from build123d import *

# Parameters (mm, degrees)
BOSS_EXTRUDE1_DEPTH      = 4
CROQUIS3_W               = 75
CROQUIS3_H               = 20
CORTAR_EXTRUIR1_DEPTH    = 10
CROQUIS4_R               = 3.5
SALIENTE_EXTRUIR1_DEPTH  = 2
CROQUIS5_R               = 2.5
SALIENTE_EXTRUIR2_DEPTH  = 27
CORTAR_EXTRUIR3_DEPTH    = 171.194006945
REDONDEO2_R              = 2
REDONDEO3_R              = 2
REDONDEO4_R              = 2
REDONDEO5_R              = 2
REDONDEO6_R              = 2
REDONDEO7_R              = 10
CROQUIS9_R               = 1.5
CORTAR_EXTRUIR4_DEPTH    = 171.194006945
CROQUIS15_R              = 3.75
SALIENTE_EXTRUIR3_DEPTH  = 10
REDONDEO8_R              = 10
REDONDEO8_OF_SIMETR_A2_R = 10
CROQUIS16_W              = 45.868264646
CROQUIS16_H              = 20
CROQUIS16_W_2            = 25.985344102
CROQUIS16_W_3            = 31
CROQUIS16_W_4            = 32
SALIENTE_EXTRUIR5_DEPTH  = 5


# Some blends are built 0.0001 mm under size
with BuildPart() as part:
    # Sketch1 → Boss-Extrude1 (new body)
    with BuildSketch(Plane(origin=(0, 0, 0), x_dir=(1, 0, 0), z_dir=(0, 1, 0))):
        with BuildLine():
            Line((70, 75), (150, 75))
            Line((150, 75), (150, 65))
            Line((150, 65), (150, -30))
            Line((150, -30), (150, -75))
            Line((150, -75), (70, -75))
            Line((70, -75), (-140, -75))
            ThreePointArc((-140, -75), (-147.071067812, -72.071067812), (-150, -65))
            Line((-150, -65), (-150, 65))
            ThreePointArc((-150, 65), (-147.071067812, 72.071067812), (-140, 75))
            Line((-140, 75), (70, 75))
        make_face()
    extrude(amount=BOSS_EXTRUDE1_DEPTH)

    # Croquis3 → Cortar-Extruir1 (cut)
    with BuildSketch(Plane(origin=(0, 4, 0), x_dir=(1, 0, 0), z_dir=(0, 1, 0))):
        with Locations((-102.5, 65)):
            Rectangle(CROQUIS3_W, CROQUIS3_H)
        with Locations((-102.5, -65)):
            Rectangle(CROQUIS3_W, CROQUIS3_H)
        Polygon((47.925951559, -36.159033642), (16.439774713, -75), (143.560225287, -75), (112.074048441, -36.159033642), (102.074048441, -36.159033642), (85, -50), (75, -50), (57.925951559, -36.159033642), align=None)
        Polygon((143.560225287, 75), (16.439774713, 75), (47.925951559, 36.159033642), (57.925951559, 36.159033642), (75, 50), (85, 50), (102.074048441, 36.159033642), (112.074048441, 36.159033642), align=None)
    cortar_extruir1 = extrude(amount=-CORTAR_EXTRUIR1_DEPTH, mode=Mode.SUBTRACT)

    # Croquis4 → Saliente-Extruir1 (add)
    with BuildSketch(Plane(origin=(0, 4, 0), x_dir=(1, 0, 0), z_dir=(0, 1, 0))):
        with Locations(Location((80, 42, 0), (0, 0, 270))):
            Circle(CROQUIS4_R)
        with Locations(Location((80, -42, 0), (0, 0, 90))):
            Circle(CROQUIS4_R)
    extrude(amount=SALIENTE_EXTRUIR1_DEPTH)

    # Croquis5 → Saliente-Extruir2 (add)
    with BuildSketch(Plane(origin=(0, 6, 0), x_dir=(1, 0, 0), z_dir=(0, 1, 0))):
        with Locations(Location((80, 42, 0), (0, 0, 270))):
            Circle(CROQUIS5_R)
        with Locations(Location((80, -42, 0), (0, 0, 90))):
            Circle(CROQUIS5_R)
    extrude(amount=SALIENTE_EXTRUIR2_DEPTH)

    # Croquis7 → Cortar-Extruir3 (cut, through all)
    with BuildSketch(Plane(origin=(0, 4, 0), x_dir=(1, 0, 0), z_dir=(0, 1, 0))):
        Polygon((57.925951559, 36.159033642), (48.662122101, 28.38575776), (40.074307196, 28.38575776), (16.439774713, 75), align=None)
        Polygon((16.439774713, -75), (57.925951559, -36.159033642), (48.662122101, -28.38575776), (40.074307196, -28.38575776), align=None)
        Polygon((143.560225287, 75), (102.074048441, 36.159033642), (111.337877899, 28.38575776), (119.925692804, 28.38575776), align=None)
        Polygon((102.074048441, -36.159033642), (111.337877899, -28.38575776), (119.925692804, -28.38575776), (143.560225287, -75), align=None)
    extrude(amount=-CORTAR_EXTRUIR3_DEPTH, mode=Mode.SUBTRACT)

    # Redondeo2
    redondeo2_edges = [part.edges().sort_by_distance(p)[0] for p in [
        (80, 4, -45.5),
    ]]
    fillet(redondeo2_edges, radius=REDONDEO2_R - 0.0001)  # a hair under: the kernel refuses the full size

    # Redondeo3
    # the kernel refuses this fillet: 2 mm, written as the material it adds along each edge
    with BuildSketch(Plane(origin=(80, 6, -42), x_dir=(0, 0, 1), z_dir=(-1, 0, 0))) as redondeo3_piece_1:
        with BuildLine():
            CenterArc((4.5, 1.732050808), REDONDEO3_R, 180, 60)
            Line((2.5, 1.732050808), (2.46, 1.732050808))
            Line((2.46, 1.732050808), (2.46, 0))
            Line((2.46, 0), (2.5, -0.04))
            ThreePointArc((2.5, -0.04), (3, -0.04), (3.48, -0.034641016))
            Line((3.48, -0.034641016), (3.5, 0))
        make_face()
    revolve(axis=Axis((80, 6, -42), (0, 1, 0)))

    # Redondeo4
    redondeo4_edges = [part.edges().sort_by_distance(p)[0] for p in [
        (80, 6, -45.5),
    ]]
    fillet(redondeo4_edges, radius=REDONDEO4_R)

    # Redondeo5
    # the kernel refuses this fillet: 2 mm, written as the material it adds along each edge
    with BuildSketch(Plane(origin=(80, 4, 42), x_dir=(0, 0, -1), z_dir=(1, 0, 0))) as redondeo5_piece_1:
        with BuildLine():
            CenterArc((3.5 + REDONDEO5_R, REDONDEO5_R), REDONDEO5_R, 180, 90)
            Line((3.5, REDONDEO5_R), (3.5 - REDONDEO5_R * 0.02, REDONDEO5_R))
            Line((3.5 - REDONDEO5_R * 0.02, REDONDEO5_R), (3.5 - REDONDEO5_R * 0.02, -REDONDEO5_R * 0.02))
            Line((3.5 - REDONDEO5_R * 0.02, -REDONDEO5_R * 0.02), (3.5 + REDONDEO5_R, -REDONDEO5_R * 0.02))
            Line((3.5 + REDONDEO5_R, -REDONDEO5_R * 0.02), (3.5 + REDONDEO5_R, 0))
        make_face()
    revolve(axis=Axis((80, 4, 42), (0, 1, 0)))
    with BuildSketch(Plane(origin=(80, 6, 42), x_dir=(0, 0, -1), z_dir=(1, 0, 0))) as redondeo5_piece_2:
        with BuildLine():
            CenterArc((4.5, 1.732050808), REDONDEO5_R, 180, 60)
            Line((2.5, 1.732050808), (2.46, 1.732050808))
            Line((2.46, 1.732050808), (2.46, 0))
            Line((2.46, 0), (2.5, -0.04))
            ThreePointArc((2.5, -0.04), (3, -0.04), (3.48, -0.034641016))
            Line((3.48, -0.034641016), (3.5, 0))
        make_face()
    revolve(axis=Axis((80, 6, 42), (0, 1, 0)))

    # Redondeo6
    redondeo6_edges = [part.edges().sort_by_distance(p)[0] for p in [
        (80, 6, 45.5),
    ]]
    fillet(redondeo6_edges, radius=REDONDEO6_R)

    # Redondeo7
    # the kernel refuses this fillet: 10 mm, written as the material it adds along each edge
    with BuildSketch(Plane(origin=(40.074307196, 4, 28.38575776), x_dir=(-0.4522182722164984, 0, 0.8919073013904107), z_dir=(0, -1, 0)), Plane(origin=(119.925692804, 4, 28.38575776), x_dir=(-1, 0, 0), z_dir=(0, -1, 0))) as redondeo7_piece_1:
        with BuildLine():
            CenterArc((REDONDEO7_R * 0.614168901779, -REDONDEO7_R), REDONDEO7_R, 90, 63.113904691)
            Line((-REDONDEO7_R * 0.277738399612, -REDONDEO7_R * 0.547781727784), (0, 0))
            Line((0, 0), (REDONDEO7_R * 0.614168901779, 0))
        make_face()
    extrude(amount=4)
    with BuildSketch(Plane(origin=(48.662122101, 4, 28.38575776), x_dir=(-1, 0, 0), z_dir=(0, -1, 0)), Plane(origin=(111.337877899, 4, 28.38575776), x_dir=(-0.7660444431189768, 0, 0.6427876096865409), z_dir=(0, -1, 0))) as redondeo7_piece_2:
        with BuildLine():
            CenterArc((REDONDEO7_R * 0.363970234266, -REDONDEO7_R), REDONDEO7_R, 90, 40)
            Line((-REDONDEO7_R * 0.27881737542, -REDONDEO7_R * 0.233955556881), (0, 0))
            Line((0, 0), (REDONDEO7_R * 0.363970234266, 0))
        make_face()
    extrude(amount=4)
    with BuildSketch(Plane(origin=(40.074307196, 4, -28.38575776), x_dir=(-0.4522182722164984, 0, -0.8919073013904107), z_dir=(0, -1, 0)), Plane(origin=(119.925692804, 4, -28.38575776), x_dir=(-1, 0, 0), z_dir=(0, -1, 0))) as redondeo7_piece_3:
        with BuildLine():
            CenterArc((REDONDEO7_R * 0.614168901779, REDONDEO7_R), REDONDEO7_R, 206.886095309, 63.113904691)
            Line((-REDONDEO7_R * 0.277738399612, REDONDEO7_R * 0.547781727784), (0, 0))
            Line((0, 0), (REDONDEO7_R * 0.614168901779, 0))
        make_face()
    extrude(amount=4)
    with BuildSketch(Plane(origin=(48.662122101, 4, -28.38575776), x_dir=(-1, 0, 0), z_dir=(0, -1, 0)), Plane(origin=(111.337877899, 4, -28.38575776), x_dir=(-0.7660444431189768, 0, -0.6427876096865409), z_dir=(0, -1, 0))) as redondeo7_piece_4:
        with BuildLine():
            CenterArc((REDONDEO7_R * 0.363970234266, REDONDEO7_R), REDONDEO7_R, 230, 40)
            Line((-REDONDEO7_R * 0.27881737542, REDONDEO7_R * 0.233955556881), (0, 0))
            Line((0, 0), (REDONDEO7_R * 0.363970234266, 0))
        make_face()
    extrude(amount=4)

    # Croquis9 → Cortar-Extruir4 (cut, through all)
    with BuildSketch(Plane(origin=(0, 4, 0), x_dir=(1, 0, 0), z_dir=(0, 1, 0))):
        with Locations(Location((-107.59, 25.23, 0), (0, 0, 270))):
            Circle(CROQUIS9_R)
        with Locations(Location((-79.79, 25.33, 0), (0, 0, 270))):
            Circle(CROQUIS9_R)
        with Locations(Location((-79.79, -22.45, 0), (0, 0, 270))):
            Circle(CROQUIS9_R)
        with Locations(Location((-107.59, -22.57, 0), (0, 0, 270))):
            Circle(CROQUIS9_R)
    extrude(amount=-CORTAR_EXTRUIR4_DEPTH, mode=Mode.SUBTRACT)

    # Croquis15 → Saliente-Extruir3 (add)
    with BuildSketch(Plane(origin=(0, 0, -55), x_dir=(-1, 0, 0), z_dir=(0, 0, -1))):
        with BuildLine():
            Line((89.459684655, 4), (89.459684655, 18.25))
            ThreePointArc((89.459684655, 18.25), (102.19671333, 30.27014077), (113.459684655, 16.858908145))
            Line((113.459684655, 16.858908145), (113.459684655, 4))
            Line((113.459684655, 4), (89.459684655, 4))
        make_face()
        with Locations((101.5, 18.25)):
            Circle(CROQUIS15_R, mode=Mode.SUBTRACT)
    saliente_extruir3 = extrude(amount=-SALIENTE_EXTRUIR3_DEPTH)

    # Redondeo8
    redondeo8_edges = [part.edges().sort_by_distance(p)[0] for p in [
        (-113.459684655, 4, -50),
        (-89.459684655, 4, -50),
        (-101.459684655, 4, -45),
    ]]
    fillet(redondeo8_edges, radius=REDONDEO8_R)

    # Simetría2: Cortar-Extruir1, Saliente-Extruir3 across plane
    add(cortar_extruir1.mirror(Plane.XY), mode=Mode.SUBTRACT)
    add(saliente_extruir3.mirror(Plane.XY))

    # Redondeo8 of Simetría2
    redondeo8_of_simetr_a2_edges = [part.edges().sort_by_distance(p)[0] for p in [
        (-113.459684655, 4, 50),
        (-89.459684655, 4, 50),
        (-101.459684655, 4, 45),
    ]]
    fillet(redondeo8_of_simetr_a2_edges, radius=REDONDEO8_OF_SIMETR_A2_R)

    # Croquis16 → Saliente-Extruir5 (add)
    with BuildSketch(Plane.XZ):
        Polygon((-94.131735354, 47.5), (-94.131735354, 14), (-140, 14), (-140, 47.5), (-144, 47.5), (-144, -47.5), (-140, -47.5), (-140, -14), (-94.131735354, -14), (-94.131735354, -47.5), (-90.131735354, -47.5), (-90.131735354, -14), (-44.263470708, -14), (-44.263470708, -47.5), (-40.263470708, -47.5), (-40.263470708, -14), (5.604793938, -14), (5.604793938, -47.5), (9.604793938, -47.5), (9.604793938, -14), (40.604793938, -14), (40.604793938, -22.5), (44.604793938, -22.5), (44.604793938, -14), (76.604793938, -14), (76.604793938, -22.5), (80.604793938, -22.5), (80.604793938, -14), (112.604793938, -14), (112.604793938, -22.5), (116.604793938, -22.5), (116.604793938, -14), (142.59013804, -14), (142.59013804, -67.5), (146.59013804, -67.5), (146.59013804, -14), (146.59013804, 10), (146.59013804, 14), (146.59013804, 67.5), (142.59013804, 67.5), (142.59013804, 14), (116.604793938, 14), (116.604793938, 22.5), (112.604793938, 22.5), (112.604793938, 14), (80.604793938, 14), (80.604793938, 22.5), (76.604793938, 22.5), (76.604793938, 14), (44.604793938, 14), (44.604793938, 22.5), (40.604793938, 22.5), (40.604793938, 14), (9.604793938, 14), (9.604793938, 47.5), (5.604793938, 47.5), (5.604793938, 14), (-40.263470708, 14), (-40.263470708, 47.5), (-44.263470708, 47.5), (-44.263470708, 14), (-90.131735354, 14), (-90.131735354, 47.5), align=None)
        with Locations((-117.065867677, 0)):
            Rectangle(CROQUIS16_W, CROQUIS16_H, mode=Mode.SUBTRACT)
        with Locations((129.597465989, 0)):
            Rectangle(CROQUIS16_W_2, CROQUIS16_H, mode=Mode.SUBTRACT)
        with Locations((25.104793938, 0)):
            Rectangle(CROQUIS16_W_3, CROQUIS16_H, mode=Mode.SUBTRACT)
        with Locations((60.604793938, 0)):
            Rectangle(CROQUIS16_W_4, CROQUIS16_H, mode=Mode.SUBTRACT)
        with Locations((96.604793938, 0)):
            Rectangle(CROQUIS16_W_4, CROQUIS16_H, mode=Mode.SUBTRACT)
        with Locations((-17.329338385, 0)):
            Rectangle(CROQUIS16_W, CROQUIS16_H, mode=Mode.SUBTRACT)
        with Locations((-67.197603031, 0)):
            Rectangle(CROQUIS16_W, CROQUIS16_H, mode=Mode.SUBTRACT)
    extrude(amount=SALIENTE_EXTRUIR5_DEPTH)


solid = part.part
Design review of the part built by this model. Coordinates are the model's own, in mm. A direction names the side the tool comes from. Round coordinates to 2 decimals unless told otherwise and drop trailing zeros. Write each loop counter-clockwise with the first axis right and the second up, starting at its lowest first coordinate (ties: lowest second). Pieces come first, ordered by that corner, then holes. Notation, with made-up numbers: (40.5, 30) - (69.5, 30) arc R5 ccw to (69.5, 35) - close; hole circle Ø8 at (1, -36.75). An arc over 180 degrees is marked (long way). Return JSON: item names as keys, results as strings. Group by question number.
Item 1: We need section B-B on y = 27.5. Write out the cut boundary in (x, z), and give its area (3 significant figures).
Item 2: The part is to be moulded in two halves that separate along Z. For faces 5 (the face through (-146.99, 1.97, 72.15)), 6 (the face through (96, 0, 0)), 7 (the face through (-104.964, 16.814, -50.07)), 8 (the face through (-117, 0, 0)), say which applies: pulls with the +Z half, pulls with the -Z half, needs draft (parallel to the pull), parting line crosses it, or undercut.
Item 3: For probe 1 along X at (y, z) = (1.4, 22.45); probe 2 along Z at (x, y) = (-79.79, 1.7); probe 3 along Y at (x, z) = (-101, -51), list the stretches that pass through material, from the lowest coordinate up. Write a range as [from, to].
Item 4: We need section A-A on x = -101.5. Write out the cut boundary in (y, z).
Item 5: Machinability: for faces 1 (the face through (-101.7, 22.3, 45)), 2 (the face through (-68, 0, 0)), 3 (the face through (-104.964, 16.814, 50.07)), 4 (the face through (66.34, 2.03, -42.98)), which of the approach directions +Z, -Z, +X, -X, +Y, -Y give a long, thin tool a straight path to every point of the face, cutting with its end or side? Answer none if there is none.
Item 6: We need section C-C on x = -69.5. Write out the cut boundary in (y, z).
Item 7: Insertion check: P1, Ø5, axis at x = 101, z = 38, coming from the +Y side; P2, Ø1.5, axis at x = -117.5, y = -2, coming from the +Z side; P3, Ø5, axis at x = -102.5, y = 7, coming from the +Z side. Each pin has a flat end and moves straight along its axis. Give the tip position at first contact, or say it passes through.
Model answer:
{
 "1": {"outline": "(-109.21, -55) - (-93.79, -55) - (-93.79, -45) - (-109.21, -45) - close; (-109.21, 45) - (-93.79, 45) - (-93.79, 55) - (-109.21, 55) - close; circle Ø5 at (80, -42); circle Ø5 at (80, 42)", "area": "348 mm²"},
 "2": {"face 5": "pulls with the +Z half", "face 6": "undercut", "face 7": "needs draft", "face 8": "undercut"},
 "3": {"probe 1": "x = [-150, -109.09], [-106.09, -81.29], [-78.29, 150]", "probe 2": "z = [-55, -26.83], [-23.83, 20.95], [23.95, 55]", "probe 3": "y = [0, 14.53], [21.97, 30.28]"},
 "4": {"outline": "(-5, -14) - (0, -14) - (0, -55) - (14.5, -55) - (14.5, -45) - (14, -45) arc R10 cw to (4, -35) - (4, 35) arc R10 cw to (14, 45) - (14.5, 45) - (14.5, 55) - (0, 55) - (0, 14) - (-5, 14) - (-5, 10) - (0, 10) - (0, -10) - (-5, -10) - close; (22, -55) - (30.29, -55) - (30.29, -45) - (22, -45) - close; (22, 45) - (30.29, 45) - (30.29, 55) - (22, 55) - close"},
 "5": {"face 1": "+X, -X, +Y", "face 2": "-Y", "face 3": "+Z, -Z", "face 4": "-Z, +Y, -Y"},
 "6": {"outline": "(-5, -14) - (0, -14) - (0, -55) - (4, -55) - (4, 55) - (0, 55) - (0, 14) - (-5, 14) - (-5, 10) - (0, 10) - (0, -10) - (-5, -10) - close"},
 "7": {"P1": "stops at y = 4", "P2": "stops at z = 14", "P3": "stops at z = 55"}
}
